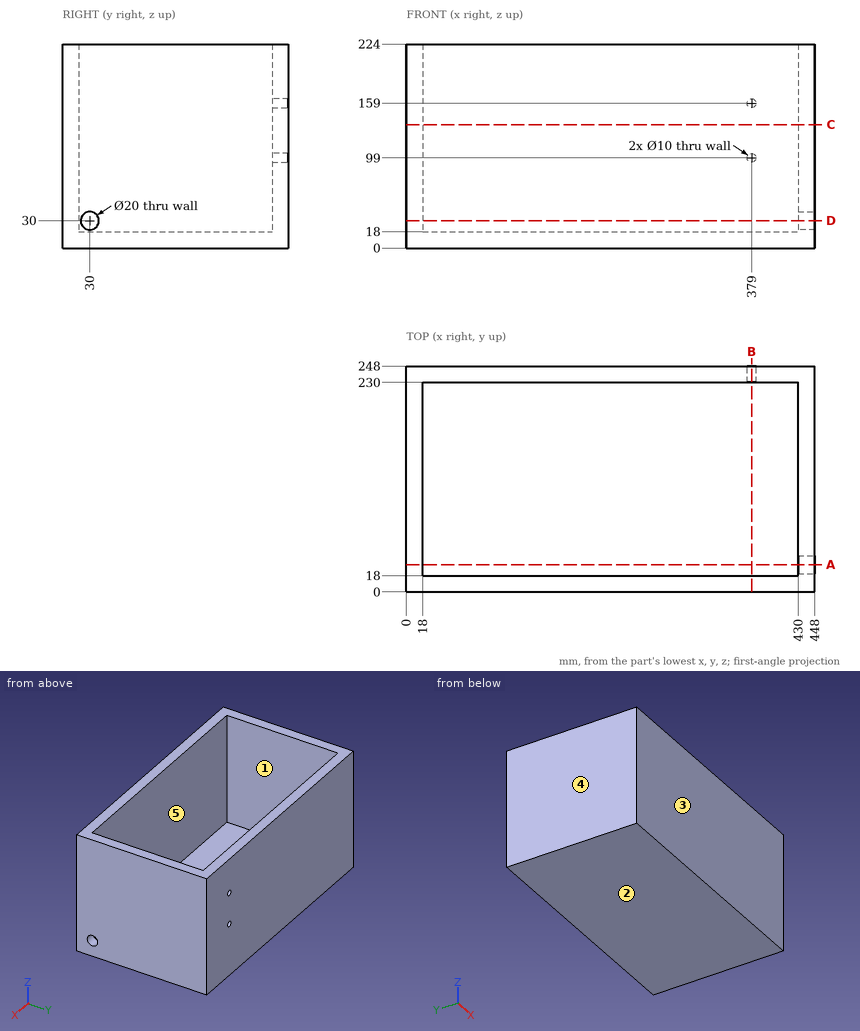
The drawing under review shows one solid part. Ordinate dimensions are in mm from its lowest x, y, z. A direction names the side the tool comes from. Give positions to 0.01 mm unless a question says otherwise; leave off trailing zeros. Loops run counter-clockwise (first coordinate to the right, second up) from the corner with the lowest first, then second, coordinate; pieces in that order, holes last. Notation, with made-up numbers: M 8,-16 L 44,-16 A12 ccw 44,3 Z; hole C 79.25,77 d8. An arc over 180 degrees is marked long. Return JSON: item names as keys, results as strings. Group by question number.
Item 1: We need section B-B (x = 379). Give the boundary of the cut face in (y, z), and give its area (3 significant figures).
Item 2: Tool access review of the marked faces 1 and 2: name each direction out of +Z, -Z, +X, -X, +Y, -Y from which nothing blocks a thin tool from reaching the whole face with its end or side.
Item 3: We need section D-D (z = 30). Give the boundary of the cut face in (x, y), and give its area (3 significant figures).
Item 4: We need section C-C (z = 135.5). Give the boundary of the cut face in (x, y), and give its area (3 significant figures).
Item 5: For probe 1 along Z at (x, y) = (379, 242); probe 2 along Y at (x, z) = (145.5, 22.5); probe 3 along Y at (x, z) = (440, 30), list the stretches that pass through material, from the lowest coordinate up.
Item 6: We need section A-A (y = 30). Give the boundary of the cut face in (x, z).
Item 7: Insertion check: pin 1 Ø9 at (x, z) = (379, 159) entering from +Y. The pin has a flat end and moves straight along its axis. Give the tip position at first contact, or say it passes through.
Item 8: Mouldability with a two-part tool opening along X and no side actions: class the marked faces 3, 4 and 5 as released by +X, released by -X, zero draft, split by the parting line, or undercut.
Output:
{
 "1": {"outline": "M 0,0 L 248,0 L 248,94 L 230,94 L 230,18 L 18,18 L 18,224 L 0,224 Z; M 230,104 L 248,104 L 248,154 L 230,154 Z; M 230,164 L 248,164 L 248,224 L 230,224 Z", "area": "11,500 mm^2"},
 "2": {"face 1": "+Z", "face 2": "-Z, +X, -X, +Y, -Y"},
 "3": {"outline": "M 0,0 L 448,0 L 448,20 L 430,20 L 430,18 L 18,18 L 18,230 L 430,230 L 430,40 L 448,40 L 448,248 L 0,248 Z", "area": "23,400 mm^2"},
 "4": {"outline": "M 0,0 L 448,0 L 448,248 L 0,248 Z; hole M 18,18 L 430,18 L 430,230 L 18,230 Z", "area": "23,800 mm^2"},
 "5": {"probe 1": "z = 0 to 94, 104 to 154, 164 to 224", "probe 2": "y = 0 to 18, 230 to 248", "probe 3": "y = 0 to 20, 40 to 248"},
 "6": {"outline": "M 0,0 L 448,0 L 448,20 L 430,20 L 430,18 L 18,18 L 18,224 L 0,224 Z; M 430,40 L 448,40 L 448,224 L 430,224 Z"},
 "7": {"pin 1": "stops at y = 18"},
 "8": {"face 3": "zero draft", "face 4": "released by -X", "face 5": "undercut"}
}
